from build123d import *

# Parameters (mm, degrees)
F0_R     = 6.35
F0_R_2   = 3.175
F1_DEPTH = 6.35
F2_SIZE  = 6.34999
F3_DEPTH = 6.351
F4_DEPTH = 6.35
F5_R     = 0.7939024


# Not quite as in the source:
# - a fillet or chamfer is up to 0.001 mm smaller than in the source, because OpenCascade refuses the exact size


with BuildPart() as f1:
    # F0 (on Top) → F1 (new body)
    with BuildSketch(Plane.XY):
        Polygon((-14.2875, 15.875), (-23.8125, 15.875), (-23.8125, 7.9375), (-31.75, 7.9375), (-31.75, -7.9375), (-23.8125, -7.9375), (-23.8125, -15.875), (-14.2875, -15.875), (-14.2875, -7.9375), (-6.35, -7.9375), (-6.35, -15.875), (6.35, -15.875), (6.35, -7.9375), (14.2875, -7.9375), (14.2875, -15.875), (23.8125, -15.875), (23.8125, -7.9375), (31.75, -7.9375), (31.75, 7.9375), (23.8125, 7.9375), (23.8125, 15.875), (14.2875, 15.875), (14.2875, 7.9375), (6.35, 7.9375), (6.35, 15.875), (-6.35, 15.875), (-6.35, 7.9375), (-14.2875, 7.9375), align=None)
        with Locations((-19.05, 0)):
            Circle(F0_R, mode=Mode.SUBTRACT)
        with Locations((19.05, 0)):
            Circle(F0_R, mode=Mode.SUBTRACT)
        with Locations((-19.05, 0)):
            Circle(F0_R)
        with Locations((-19.05, 0)):
            Circle(F0_R_2, mode=Mode.SUBTRACT)
        with Locations((19.05, 0)):
            Circle(F0_R)
        with Locations((19.05, 0)):
            Circle(F0_R_2, mode=Mode.SUBTRACT)
        with Locations((-19.05, 0)):
            Circle(F0_R_2)
        with Locations((19.05, 0)):
            Circle(F0_R_2)
        Polygon((-23.8125, 7.9375), (-31.75, 15.875), (-31.75, 7.9375), align=None)
        Polygon((-23.8125, 15.875), (-31.75, 15.875), (-23.8125, 7.9375), align=None)
        Polygon((-6.35, 15.875), (-14.2875, 15.875), (-14.2875, 7.9375), align=None)
        Polygon((-6.35, 7.9375), (-6.35, 15.875), (-14.2875, 7.9375), align=None)
        Polygon((14.2875, 7.9375), (6.35, 15.875), (6.35, 7.9375), align=None)
        Polygon((14.2875, 15.875), (6.35, 15.875), (14.2875, 7.9375), align=None)
        Polygon((31.75, 15.875), (23.8125, 15.875), (23.8125, 7.9375), align=None)
        Polygon((31.75, 7.9375), (31.75, 15.875), (23.8125, 7.9375), align=None)
        Polygon((31.75, -15.875), (31.75, -7.9375), (23.8125, -7.9375), align=None)
        Polygon((23.8125, -7.9375), (23.8125, -15.875), (31.75, -15.875), align=None)
        Polygon((14.2875, -7.9375), (6.35, -15.875), (14.2875, -15.875), align=None)
        Polygon((6.35, -7.9375), (6.35, -15.875), (14.2875, -7.9375), align=None)
        Polygon((-14.2875, -7.9375), (-6.35, -15.875), (-6.35, -7.9375), align=None)
        Polygon((-14.2875, -7.9375), (-14.2875, -15.875), (-6.35, -15.875), align=None)
        Polygon((-23.8125, -7.9375), (-31.75, -15.875), (-23.8125, -15.875), align=None)
        Polygon((-23.8125, -7.9375), (-31.75, -7.9375), (-31.75, -15.875), align=None)
    extrude(amount=F1_DEPTH)

    # F2 (size 6.35 in the source; OpenCascade refuses exactly that, so slightly less here)
    f2_edges = [f1.edges().sort_by_distance(p)[0] for p in [
        (31.75, 0, 6.35),
        (0, 15.875, 6.35),
        (-31.75, 0, 6.35),
        (0, -15.875, 6.35),
    ]]
    chamfer(f2_edges, length=F2_SIZE)

    # F0 (on Top) → F3 (cut, through all)
    with BuildSketch(Plane.XY):
        with Locations((-19.05, 0)):
            Circle(F0_R_2)
        with Locations((19.05, 0)):
            Circle(F0_R_2)
    extrude(amount=F3_DEPTH, mode=Mode.SUBTRACT)

    # F0 (on Top) → F4 (join)
    with BuildSketch(Plane.XY):
        with Locations((-19.05, 0)):
            Circle(F0_R)
        with Locations((-19.05, 0)):
            Circle(F0_R_2, mode=Mode.SUBTRACT)
        with Locations((19.05, 0)):
            Circle(F0_R)
        with Locations((19.05, 0)):
            Circle(F0_R_2, mode=Mode.SUBTRACT)
    extrude(amount=-F4_DEPTH)

    # F5
    f5_edges = [f1.edges().sort_by_distance(p)[0] for p in [
        (-25.4, 0, -6.35),
        (12.7, 0, -6.35),
    ]]
    fillet(f5_edges, radius=F5_R)


solid = f1.part
Model file for the job. Use its own axes, mm. A direction names the side the tool comes from. Coordinates: 2 decimals unless noted, no trailing zeros. Order: outer loops, then holes, each group sorted by start corner. A loop starts at its lowest first (then second) coordinate and runs counter-clockwise, first axis right, second up. Notation, with made-up numbers: (84, 53) -> (104, 53) arc R20 ccw to (104, 87) -> close; hole circle Ø1 at (85, 26.25). An arc over 180 degrees is marked (long way). Return JSON: item names as keys, results as strings. Group by question number.
Item 1: Saw through at A-A on y = 0. State how many separate pieces and enclosed holes the cut face has, then the cut area to 3 significant figures.
Item 2: Wall check: line 1 along Y through (x, z) = (19.05, -2.5) (3 decimals); line 2 along X through (y, z) = (1.5, -2.5); line 3 along X through (y, z) = (0, 3.75) (3 decimals). Give the ranges that are in metal, low to high. Write a range as [from, to].
Item 3: Tool access for faces 4 (the cylindrical face through (-24.09, -3.86, -2.74)), 5 (the flat face through (-0.444, -12.656, 3.219)): list every direction of +Z, -Z, +X, -X, +Y, -Y with a clear straight run to the whole face (end or side of a thin tool).
Item 4: Flat gauge pins, fed straight in: P1, Ø4, axis at y = -5, z = -2.5, coming from the -X side; P2, Ø5, axis at x = 0.5, y = 12, coming from the -Z side; P3, Ø1.5, axis at y = -3, z = 3.5, coming from the -X side. Where does each tip first touch, or does it go through?
Item 5: Pull direction Z, two halves, no side cores. Call faces 1 (the flat face through (21.4, -2.4, -6.35)), 2 (the cylindrical face through (15.88, 0.14, 0.09)), 3 (the flat face through (0, 0, 6.35)): pulls with the +Z half, pulls with the -Z half, needs draft (parallel to the pull), parting line crosses it, or undercut.
Item 6: Saw through at C-C on z = -3. Write the cut outline in (x, y) (3 decimals).
Values found:
{
 "1": {"separate pieces": "3", "enclosed holes": "0", "area": "362 mm2"},
 "2": {"line 1": "y = [-6.35, -3.175], [3.175, 6.35]", "line 2": "x = [-25.22, -21.85], [-16.25, -12.88], [12.88, 16.25], [21.85, 25.22]", "line 3": "x = [-28, -22.225], [-15.875, 15.875], [22.225, 28]"},
 "3": {"face 4": "-Z", "face 5": "+Z, +X, -X, -Y"},
 "4": {"P1": "stops at x = -24.65", "P2": "stops at z = 0", "P3": "stops at x = -29"},
 "5": {"face 1": "pulls with the -Z half", "face 2": "needs draft", "face 3": "pulls with the +Z half"},
 "6": {"outline": "circle Ø12.7 at (-19.05, 0); circle Ø12.7 at (19.05, 0); hole circle Ø6.35 at (-19.05, 0); hole circle Ø6.35 at (19.05, 0)"}
}
